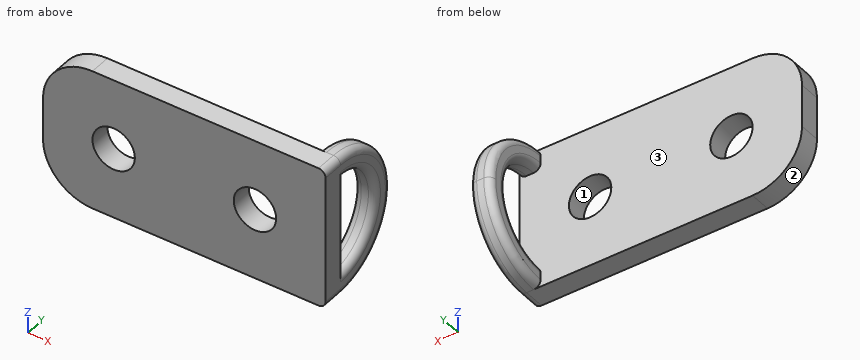
from build123d import *

# Parameters (mm, degrees)
SKETCH1_R           = 3
BOSS_EXTRUDE1_DEPTH = 3
SKETCH2_W           = 3
SKETCH2_H           = 20
BOSS_EXTRUDE2_DEPTH = 10
FILLET1_R           = 10
CUT_EXTRUDE1_DEPTH  = 45.022721406
FILLET2_R           = 1


with BuildPart() as part:
    # Sketch1 → Boss-Extrude1 (new body)
    with BuildSketch(Plane(origin=(0, 0, 0), x_dir=(1, 0, 0), z_dir=(0, 1, 0))):
        with BuildLine():
            Line((0, 0), (-33, 0))
            ThreePointArc((-33, 0), (-37.949747468, -2.050252532), (-40, -7))
            Line((-40, -7), (-40, -13))
            ThreePointArc((-40, -13), (-37.949747468, -17.949747468), (-33, -20))
            Line((-33, -20), (0, -20))
            Line((0, -20), (0, 0))
        make_face()
        with Locations(Location((-30, -10, 0), (0, 0, 270))):
            Circle(SKETCH1_R, mode=Mode.SUBTRACT)
        with Locations(Location((-10, -10, 0), (0, 0, 270))):
            Circle(SKETCH1_R, mode=Mode.SUBTRACT)
    extrude(amount=BOSS_EXTRUDE1_DEPTH)

    # Sketch2 → Boss-Extrude2 (add)
    with BuildSketch(Plane(origin=(0, 3, 0), x_dir=(1, 0, 0), z_dir=(0, 1, 0))):
        with Locations((-1.5, -10)):
            Rectangle(SKETCH2_W, SKETCH2_H)
    extrude(amount=BOSS_EXTRUDE2_DEPTH)

    # Fillet1
    fillet1_edges = [part.edges().sort_by_distance(p)[0] for p in [
        (-1.5, 13, 0),
        (-1.5, 13, 20),
    ]]
    fillet(fillet1_edges, radius=FILLET1_R - 0.0001)  # a hair under: the kernel refuses the full size

    # Sketch3 → Cut-Extrude1 (cut, through all)
    with BuildSketch(Plane.ZY.offset(3)):
        with BuildLine():
            Line((3, 3), (17, 3))
            ThreePointArc((17, 3), (10, 10), (3, 3))
        make_face()
    extrude(amount=-CUT_EXTRUDE1_DEPTH, mode=Mode.SUBTRACT)

    # Fillet2
    fillet2_edges = [part.edges().sort_by_distance(p)[0] for p in [
        (-3, 10.071097101, 17.071097101),
        (-3, 10.071097101, 2.928902899),
        (0, 1.50005, 0),
        (0, 1.50005, 20),
        (0, 10.071097101, 17.071097101),
        (0, 10.071097101, 2.928902899),
        (0, 10, 10),
        (-3, 10, 10),
    ]]
    fillet(fillet2_edges, radius=FILLET2_R)


solid = part.part
Can you work these out from the model? Positions are in its coordinate system, mm. Face numbers are marked on the shaded views. Round coordinates to 2 decimals unless told otherwise and drop trailing zeros. Write each loop counter-clockwise with the first axis right and the second up, starting at its lowest first coordinate (ties: lowest second). Pieces come first, ordered by that corner, then holes. Notation, with made-up numbers: (51.25, 8.25) -> (61.25, 8.25) arc R22 ccw to (61.25, 15.25) -> close; hole circle Ø5 at (-31.75, 61.25). An arc over 180 degrees is marked (long way). Use one line per item in the form item = value. Start each with the question number.
Q1. Imagine slicing it at B-B (x = -16.5). Please give me the cut outline in (y, z).
Q2. We'd pull the mould along X, two halves only. Please class the marked faces 1, 2 and 3: +X half, -X half, draft (parallel to the pull), parting line (faces both ways), or undercut.
Q3. If I drill on probe 1 along X at (y, z) = (1.2, 10); probe 2 along Y at (x, z) = (-5.5, 2.25); probe 3 along X at (y, z) = (12, 11), over which ranges is the centre line in solid material (lowest first)? Write a range as [from, to].
Q4. Imagine slicing it at A-A (x = -32.5). Please give me the cut outline in (y, z), then the cut area to 4 significant figures.
Q5. I'm going to push flat-ended pins straight in: P1, Ø1.5, axis at x = -16.5, z = 2.5, coming from the -Y side; P2, Ø10, axis at x = -7, z = 3, coming from the +Y side; P3, Ø4, axis at x = -15, z = 3.5, coming from the +Y side; P4, Ø7, axis at y = 8, z = 10, coming from the -X side. Where does each tip first touch, or does it pass through?
Q6. Imagine slicing it at C-C (x = -37). Please give me the cut outline in (y, z).
Worked out:
q1.outline = (0, 0) -> (3, 0) -> (3, 20) -> (0, 20) -> close
q2.face_1 = undercut
q2.face_2 = -X half
q2.face_3 = draft
q3.probe_1 = [-40, -33], [-27, -13], [-7, 0]
q3.probe_2 = [0, 3]
q3.probe_3 = [-3, 0]
q4.outline = (0, 0) -> (3, 0) -> (3, 8.34) -> (0, 8.34) -> close; (0, 11.66) -> (3, 11.66) -> (3, 20) -> (0, 20) -> close
q4.area = 50.05 mm^2
q5.P1 = 0
q5.P2 = 11.64
q5.P3 = 3
q5.P4 = -3
q6.outline = (0, 1.26) -> (3, 1.26) -> (3, 18.74) -> (0, 18.74) -> close
